Here's the drawing with two shaded views (mm, measured from the low corner). I have some questions. A direction names the side the tool comes from. Round coordinates to 2 decimals unless told otherwise and drop trailing zeros. Order: outer loops, then holes, each group sorted by start corner. A loop starts at its lowest first (then second) coordinate and runs counter-clockwise, first axis right, second up. Notation, with made-up numbers: M 10.25,9 L 27.25,9 A22 cw 27.25,25 Z; hole C 49.25,-22 d8. An arc over 180 degrees is marked long. One line per question, with ' | ' between items.
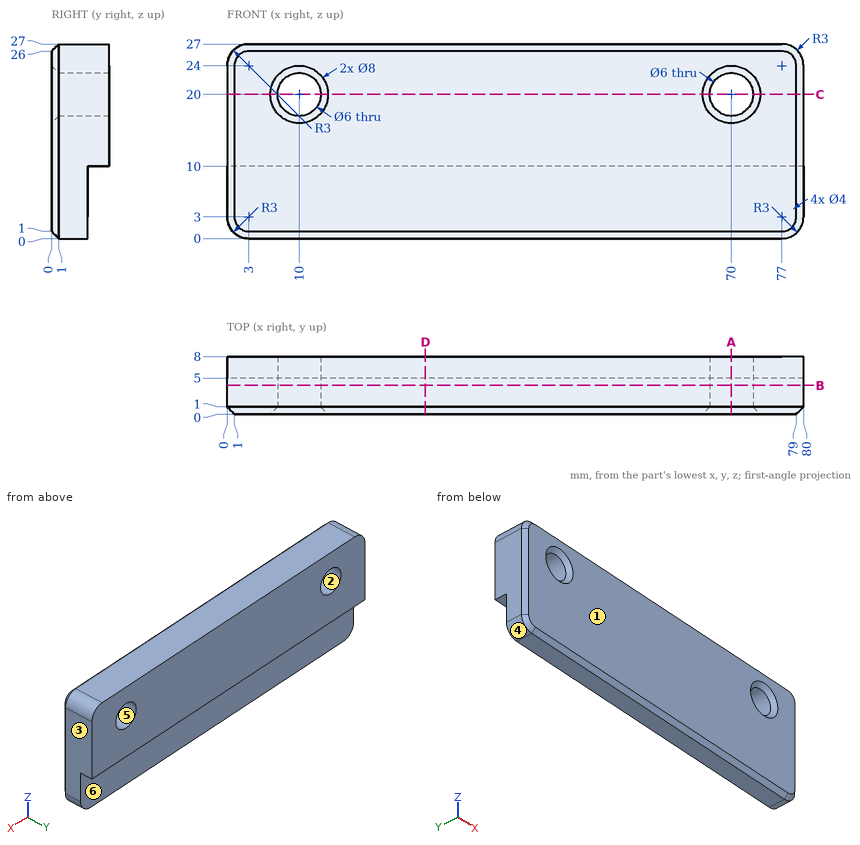
(1) Will these pins go through, and if not, where does the flat tip stop? pin 1 Ø11 at (x, z) = (31, 5.5) entering from +Y; pin 2 Ø7 at (x, z) = (10, 20) entering from -Y; pin 3 Ø1.5 at (x, y) = (38.5, 7) entering from -Z; pin 4 Ø3 at (x, z) = (8, 4.5) entering from +Y.
Final values:
pin 1: y = 8 | pin 2: y = 0.5 | pin 3: z = 10 | pin 4: y = 5
(2) If we section it at D-D on x = 27.5: Please give me the cut outline in (y, z).
Final values:
outline: M 0,1 L 1,0 L 5,0 L 5,10 L 8,10 L 8,27 L 1,27 L 0,26 Z
(3) Thinking about a two-plate mould opening in X: for the marked faces 1, 2, 3 and 4, which applies, released by +X, released by -X, zero draft, split by the parting line, or undercut?
Final values:
face 1: zero draft | face 2: undercut | face 3: released by +X | face 4: released by -X
(4) If we section it at A-A on x = 70: Please give me the cut outline in (y, z), plus the area to 3 significant figures.
Final values:
outline: M 0,1 L 1,0 L 5,0 L 5,10 L 8,10 L 8,17 L 1,17 L 0,16 Z; M 0,24 L 1,23 L 8,23 L 8,27 L 1,27 L 0,26 Z | area: 136 mm^2
(5) Please list where these lines run through material, in increasing order: probe 1 along X at (y, z) = (3, 20); probe 2 along X at (y, z) = (3.5, 17.75); probe 3 along Y at (x, z) = (6, 7). Write a range as [from, to].
Final values:
probe 1: [0, 7], [13, 67], [73, 80] | probe 2: [0, 8.02], [11.98, 68.02], [71.98, 80] | probe 3: [0, 5]
(6) If we section it at C-C on z = 20: Please give me the cut outline in (x, y).
Final values:
outline: M 0,1 L 1,0 L 6,0 L 7,1 L 7,8 L 0,8 Z; M 13,1 L 14,0 L 66,0 L 67,1 L 67,8 L 13,8 Z; M 73,1 L 74,0 L 79,0 L 80,1 L 80,8 L 73,8 Z
(7) If we section it at B-B on y = 4: Please give me the cut outline in (x, z), plus the area to 3 significant figures.
Final values:
outline: M 0,3 A3 ccw 3,0 L 77,0 A3 ccw 80,3 L 80,24 A3 ccw 77,27 L 3,27 A3 ccw 0,24 Z; hole C 10,20 d6; hole C 70,20 d6 | area: 2,100 mm^2
(8) On a 3-axis mill with a long thin cutter (end or side, diameter ignored), from which of +Z, -Z, +X, -X, +Y, -Y can I reach the whole of each face in a straight line? I mean the marked faces 5 and 6. Say none if no direction works.
Final values:
face 5: +Y, -Y | face 6: -Z, +X, -X, +Y
